from build123d import *

# Parameters (mm, degrees)
BOX006_W     = 20
BOX006_H     = 3
BOX006_DEPTH = 6
BOX005_W     = 20
BOX005_H     = 3
BOX005_DEPTH = 6
BOX004_W     = 20
BOX004_H     = 3
BOX004_DEPTH = 6
BOX003_W     = 20
BOX003_H     = 3
BOX003_DEPTH = 6
BOX002_W     = 20
BOX002_H     = 3
BOX002_DEPTH = 6
BOX001_W     = 20
BOX001_H     = 3
BOX001_DEPTH = 6
BOX_W        = 171
BOX_H        = 58
BOX_DEPTH    = 2
BOX007_W     = 3
BOX007_H     = 58
BOX007_DEPTH = 1


with BuildPart() as cube006:
    # Box006 → Box006 (new body)
    with BuildSketch(Plane(origin=(127.22, 51.5, 0), x_dir=(1, 0, 0), z_dir=(0, 0, 1))):
        with Locations((10, 1.5)):
            Rectangle(BOX006_W, BOX006_H)
    extrude(amount=BOX006_DEPTH)


with BuildPart() as cube005:
    # Box005 → Box005 (new body)
    with BuildSketch(Plane(origin=(78.15, 51.5, 0), x_dir=(1, 0, 0), z_dir=(0, 0, 1))):
        with Locations((10, 1.5)):
            Rectangle(BOX005_W, BOX005_H)
    extrude(amount=BOX005_DEPTH)


with BuildPart() as cube004:
    # Box004 → Box004 (new body)
    with BuildSketch(Plane(origin=(29.07, 51.5, 0), x_dir=(1, 0, 0), z_dir=(0, 0, 1))):
        with Locations((10, 1.5)):
            Rectangle(BOX004_W, BOX004_H)
    extrude(amount=BOX004_DEPTH)


with BuildPart() as cube003:
    # Box003 → Box003 (new body)
    with BuildSketch(Plane(origin=(127.22, 3.5, 0), x_dir=(1, 0, 0), z_dir=(0, 0, 1))):
        with Locations((10, 1.5)):
            Rectangle(BOX003_W, BOX003_H)
    extrude(amount=BOX003_DEPTH)


with BuildPart() as cube002:
    # Box002 → Box002 (new body)
    with BuildSketch(Plane(origin=(78.15, 3.5, 0), x_dir=(1, 0, 0), z_dir=(0, 0, 1))):
        with Locations((10, 1.5)):
            Rectangle(BOX002_W, BOX002_H)
    extrude(amount=BOX002_DEPTH)


with BuildPart() as cube001:
    # Box001 → Box001 (new body)
    with BuildSketch(Plane(origin=(29.07, 3.5, 0), x_dir=(1, 0, 0), z_dir=(0, 0, 1))):
        with Locations((10, 1.5)):
            Rectangle(BOX001_W, BOX001_H)
    extrude(amount=BOX001_DEPTH)


with BuildPart() as cube:
    # Box → Box (new body)
    with BuildSketch(Plane(origin=(3, 0, 0), x_dir=(1, 0, 0), z_dir=(0, 0, 1))):
        with Locations((85.5, 29)):
            Rectangle(BOX_W, BOX_H)
    extrude(amount=BOX_DEPTH)


with BuildPart() as fusion:
    # Box007 → Box007 (new body)
    with BuildSketch(Plane.XY):
        with Locations((1.5, 29)):
            Rectangle(BOX007_W, BOX007_H)
    extrude(amount=BOX007_DEPTH)

    # Fusion: union Cube006, Cube005, Cube004, Cube003, Cube002, Cube001, Cube
    add(cube006.part)
    add(cube005.part)
    add(cube004.part)
    add(cube003.part)
    add(cube002.part)
    add(cube001.part)
    add(cube.part)


solid = fusion.part
Can you work these out from the model? Positions are in its coordinate system, mm. A direction names the side the tool comes from. Round coordinates to 2 decimals unless told otherwise and drop trailing zeros. Write each loop counter-clockwise with the first axis right and the second up, starting at its lowest first coordinate (ties: lowest second). Pieces come first, ordered by that corner, then holes. Notation, with made-up numbers: (50.5, 37) -> (96.5, 37) arc R23 cw to (96.5, 70) -> close; hole circle Ø3 at (58.25, 83). An arc over 180 degrees is marked (long way). Use one line per item in the form item = value. Start each with the question number.
Q1. Imagine slicing it at D-D (x = 26). Please give me the cut outline in (y, z), then the cut area to 3 significant figures.
Q2. Imagine slicing it at A-A (z = 3.8). Please give me the cut outline in (x, y).
Q3. We'd pull the mould along X, two halves only. Please class faces 6 (the face through (29.07, 53, 4)), 7 (the face through (39, 54.5, 4)), 8 (the face through (78.15, 53, 4)), 9 (the face through (78.15, 5, 4)): +X half, -X half, draft (parallel to the pull), parting line (faces both ways), or undercut.
Q4. Which directions (+Z, -Z, +X, -X, +Y, -Y) give clear straight access to the entire face, cutting with the end or side of a thin tool? Please do faces 1 (the face through (147.22, 53, 4)), 2 (the face through (88, 3.5, 4)), 3 (the face through (137, 54.5, 4)), 4 (the face through (49.07, 53, 4)), 5 (the face through (88, 6.5, 4)).
Q5. Imagine slicing it at B-B (x = 93.5). Please give me the cut outline in (y, z), then the cut area to 3 significant figures.
Q6. Imagine slicing it at C-C (y = 33.5). Please give me the cut outline in (x, z).
Q7. I'm going to push flat-ended pins straight in: P1, Ø1.5, axis at y = 4.5, z = 5, coming from the +X side; P2, Ø3.5, axis at y = 5, z = 5, coming from the -X side; P3, Ø2, axis at x = 39.5, z = 3.5, coming from the +Y side; P4, Ø1.1, axis at y = 32, z = 1.5, coming from the -X side. Where does each tip first touch, or does it pass through?
Q8. If I drill on probe 1 along Y at (x, z) = (145, 3.7); probe 2 along X at (y, z) = (13, 1.4); probe 3 along Z at (x, y) = (60.5, 48), over which ranges is the centre line in solid material (lowest first)? Write a range as [from, to].
Worked out:
q1.outline = (0, 0) -> (58, 0) -> (58, 2) -> (0, 2) -> close
q1.area = 116 mm^2
q2.outline = (29.07, 3.5) -> (49.07, 3.5) -> (49.07, 6.5) -> (29.07, 6.5) -> close; (29.07, 51.5) -> (49.07, 51.5) -> (49.07, 54.5) -> (29.07, 54.5) -> close; (78.15, 3.5) -> (98.15, 3.5) -> (98.15, 6.5) -> (78.15, 6.5) -> close; (78.15, 51.5) -> (98.15, 51.5) -> (98.15, 54.5) -> (78.15, 54.5) -> close; (127.22, 3.5) -> (147.22, 3.5) -> (147.22, 6.5) -> (127.22, 6.5) -> close; (127.22, 51.5) -> (147.22, 51.5) -> (147.22, 54.5) -> (127.22, 54.5) -> close
q3.face_6 = -X half
q3.face_7 = draft
q3.face_8 = undercut
q3.face_9 = undercut
q4.face_1 = +Z, +X, +Y, -Y
q4.face_2 = +Z, +X, -X, -Y
q4.face_3 = +Z, +X, -X, +Y
q4.face_4 = +Z, +Y, -Y
q4.face_5 = +Z, +X, -X
q5.outline = (0, 0) -> (58, 0) -> (58, 2) -> (54.5, 2) -> (54.5, 6) -> (51.5, 6) -> (51.5, 2) -> (6.5, 2) -> (6.5, 6) -> (3.5, 6) -> (3.5, 2) -> (0, 2) -> close
q5.area = 140 mm^2
q6.outline = (0, 0) -> (174, 0) -> (174, 2) -> (3, 2) -> (3, 1) -> (0, 1) -> close
q7.P1 = 147.22
q7.P2 = 29.07
q7.P3 = 54.5
q7.P4 = 0
q8.probe_1 = [3.5, 6.5], [51.5, 54.5]
q8.probe_2 = [3, 174]
q8.probe_3 = [0, 2]
